from build123d import *

# Parameters (mm, degrees)
F1_DEPTH = 6.35
F3_D     = 5.1054
F5_D     = 5.1054
F6_D     = 28.575


with BuildPart() as f1:
    # F0 (on Top) → F1 (new body)
    with BuildSketch(Plane.XY):
        Polygon((222.605536, -187.339712), (-234.594464, 117.460288), (-234.594464, -187.339712), align=None)
    extrude(amount=F1_DEPTH)

    # F3 (through all)
    with Locations(Plane.XY.offset(6.35)):
        with Locations((-221.894464, 53.960288), (-69.494464, -174.639712), (82.905536, -174.639712), (-221.894464, -22.239712), (-221.894464, -47.639712), (-221.894464, -73.039712), (-221.894464, 28.560288), (-171.094464, -174.639712), (-221.894464, 3.160288), (108.305536, -174.639712), (-120.294464, -174.639712), (159.105536, -174.639712), (-18.694464, -174.639712), (-94.894464, -174.639712), (32.105536, -174.639712), (-221.894464, -123.839712), (-221.894464, -174.639712), (-221.894464, -98.439712), (184.505536, -174.639712), (-196.494464, -174.639712), (133.705536, -174.639712), (57.505536, -174.639712), (-145.694464, -174.639712), (-44.094464, -174.639712), (6.705536, -174.639712), (-221.894464, -149.239712), (-221.894464, 79.360288)):
            Hole(F3_D / 2)

    # F5 (through all)
    with Locations(Plane.XY.offset(6.35)):
        with Locations((-201.320464, -119.013712), (-166.268464, -119.013712), (-201.320464, -154.065712), (-166.268464, -154.065712)):
            Hole(F5_D / 2)

    # F6 (through all)
    with Locations(Plane.XY.offset(6.35)):
        with Locations((-183.794464, -136.539712)):
            Hole(F6_D / 2)


solid = f1.part
Geometry: final body of the model. Coordinates: model frame, mm. Coordinates: 2 decimals unless noted, no trailing zeros. Order: outer loops, then holes, each group sorted by start corner. A loop starts at its lowest first (then second) coordinate and runs counter-clockwise, first axis right, second up.
1) First-contact query: P1, Ø2, axis at y = -111.5, z = 5, coming from the +X side. Flat tip, straight axial feed; report the tip coordinate or a pass-through.
Result sheet:
P1: stops at x = 110.35
2) Draft query along Y for faces 1 (the flat face through (-111, -101, 0)), 2 (the flat face through (-2.794, -37.073, 3.131)), 3 (the cylindrical face through (-196.992, -142.012, 3.131)). Return one class per face: released by +Y, released by -Y, zero draft, split by the parting line, or undercut.
Result sheet:
face 1: zero draft
face 2: released by +Y
face 3: undercut
3) Section D-D (y = 46.5). Return loops of the section in (x, z).
Result sheet:
outline: (-234.59, 0) - (-128.15, 0) - (-128.15, 6.35) - (-234.59, 6.35) - close
4) Ray query, probe 1 along Y at (x, z) = (-201, 2.5); probe 2 along X at (y, z) = (-134, 5); probe 3 along Y at (x, z) = (-166, 4.25). Return the intervals inside material, ascending.
Result sheet:
probe 1: y = -187.34 to -156.6, -151.53 to -121.55, -116.48 to 95.06
probe 2: x = -234.59 to -197.85, -169.73 to 142.6
probe 3: y = -187.34 to -156.6, -151.53 to -121.55, -116.48 to 71.73
5) Section C-C (z = 1.5). Give the number of separate pieces and of enclosed holes in the cut face, then the cut area to 3 significant figures.
Result sheet:
separate pieces: 1
enclosed holes: 32
area: 68,400 mm2
6) Section B-B (y = -83.5). Return loops of the section in (x, z), then the cut area to 3 significant figures.
Result sheet:
outline: (-234.59, 0) - (66.85, 0) - (66.85, 6.35) - (-234.59, 6.35) - close
area: 1,910 mm2
7) Section A-A (x = -180). Return loops of the section in (y, z), then the cut area to 3 significant figures.
Result sheet:
outline: (-187.34, 0) - (-150.31, 0) - (-150.31, 6.35) - (-187.34, 6.35) - close; (-122.77, 0) - (81.06, 0) - (81.06, 6.35) - (-122.77, 6.35) - close
area: 1,530 mm2
